Verification items for the finished model (mm, model axes). A direction names the side the tool comes from. Round coordinates to 2 decimals unless told otherwise and drop trailing zeros. Order: outer loops, then holes, each group sorted by start corner. A loop starts at its lowest first (then second) coordinate and runs counter-clockwise, first axis right, second up. Notation, with made-up numbers: M 11,-17.5 L 59,-17.5 A20 cw 59,5.5 Z; hole C 23,23.5 d6. An arc over 180 degrees is marked long. Use CSV: the item, a comma, the result in double quotes. Start each with the question number.
Q1. Gauge pin test, flat ends, axial feed: pin 1 Ø0.9 at (x, y) = (3.5, 50.5) entering from -Z; pin 2 Ø2 at (y, z) = (19, 20.5) entering from +X; pin 3 Ø1.2 at (x, z) = (1, -32.5) entering from +Y; pin 4 Ø1.8 at (y, z) = (27.5, 26.1) entering from -X. Record the tip position at first contact, or that the pin passes through.
Q2. Sectioned sample at D-D (y = 51). Enter the section's corners in (x, z), and give its area (3 significant figures).
Q3. Sectioned sample at A-A (y = 27.5). Enter the section's corners in (x, z), and give its area (4 significant figures).
Q4. Scan lines: line 1 (Y direction, x = 0.95, z = -26.1); line 2 (Z direction, x = 0.75, y = 27); line 3 (Z direction, x = 6.5, y = 44). Record each from-to range of solid material in increasing order.
Q5. Sectioned sample at B-B (z = 26.1). Enter the section's corners in (x, y).
Q6. Set-up check for faces 1 (the face through (6, 7, 18.8)), 2 (the face through (3, 48, -27.1)), 3 (the face through (1, 14.5, -33)): record each of +Z, -Z, +X, -X, +Y, -Y from which the full face is reachable in a straight line by a thin tool's end or side.
Q7. Mould release check, pull along Z, two halves, no side actions. Record for faces 4 (the face through (1, 40.5, -33)), 5 (the face through (2.5, 27, 1)), 6 (the face through (3, 7, 27.1)): +Z half, -Z half, draft (parallel to the pull), parting line (faces both ways), or undercut.
Q8. Sectioned sample at C-C (x = 5.25). Enter the section's corners in (y, z), and give its area (3 significant figures).
Autodesk Inventor part; units mm, degrees
ref_plane "YZ Plane" through (0, 0, 0) normal (1, 0, 0) x (0, 1, 0)
ref_plane "XZ Plane" through (0, 0, 0) normal (0, 1, 0) x (-1, 0, 0)
ref_plane "XY Plane" through (0, 0, 0) normal (0, 0, 1) x (1, 0, 0)
sketch "Sketch1" plane through (0, 0, 0) normal (0, 1, 0) x (-1, 0, 0)
  line L0 (0, 27.1) -> (0, -27.1)
  line L1 (0, 27.1) -> (-6.8, 27.1)
  line L2 (-6.8, 27.1) -> (-6.8, 18.8)
  line L3 (-6.8, 18.8) -> (-4.3, 18.8)
  line L4 (-4.3, 18.8) -> (-4.3, 24.6)
  line L5 (-4.3, 24.6) -> (-2.5, 24.6)
  line L6 (-2.5, 24.6) -> (-2.5, 0)
  line L7 (0, -27.1) -> (-6.8, -27.1)
  line L8 (-6.8, -27.1) -> (-6.8, -18.8)
  line L9 (-6.8, -18.8) -> (-4.3, -18.8)
  line L10 (-4.3, -18.8) -> (-4.3, -24.6)
  line L11 (-4.3, -24.6) -> (-2.5, -24.6)
  line L12 (-2.5, -24.6) -> (-2.5, 0)
  point P0 (0, 0)
  dimension "d0" = 54.2
  dimension "d1" = 6.8
  dimension "d2" = 8.3
  dimension "d3" = 2.5
  dimension "d4" = 5.8
  dimension "d5" = 1.8
  dimension "d6" = 8.3
  dimension "d7" = 5.8
extrude "Extrusion1" add sketch "Sketch1" along normal blind 14.5
sketch "Sketch2" plane through (0, 14.5, 0) normal (0, 1, 0) x (1, 0, 0)
  line L0 (2.5, -24.6) -> (2.5, 24.6)
  line L1 (2.5, 0) -> (2.5, 39.5)
  line L2 (2.5, 39.5) -> (0, 39.5)
  line L3 (0, 39.5) -> (0, 0)
  line L4 (0, 0) -> (0, -39.5)
  line L5 (0, 27.1) -> (0, -27.1)
  line L6 (0, -39.5) -> (2.5, -39.5)
  line L7 (2.5, -39.5) -> (2.5, 0)
  dimension "d10" = 39.5
  dimension "d11" = 39.5
extrude "Extrusion2" add sketch "Sketch2" along normal blind 26
sketch "Sketch3" plane through (0, 40.5, 0) normal (0, 1, 0) x (1, 0, 0)
  line L0 (2.5, -24.6) -> (2.5, 24.6)
  line L1 (2.5, 0) -> (2.5, 24.6558)
  line L2 (0, 27.1) -> (0, -27.1)
  line L3 (4.3, -24.6) -> (2.5, -24.6)
  line L4 (6.8, -18.8) -> (4.3, -18.8)
  line L5 (4.3, -24.6) -> (4.3, -18.8)
  line L6 (4.3, -18.8) -> (6.8, -18.8)
  line L7 (6.8, -18.8) -> (6.8, -27.1)
  line L8 (6.8, -27.1) -> (2.5, -27.1)
  line L9 (2.5, 0) -> (2.5, 24.6558)
  line L10 (2.5, 24.6) -> (4.3, 24.6)
  line L11 (4.3, 18.8) -> (6.8, 18.8)
  line L12 (4.3, 24.6) -> (4.3, 18.8)
  line L13 (4.3, 18.8) -> (6.8, 18.8)
  line L14 (6.8, 18.8) -> (6.8, 27.1)
  line L15 (6.8, 27.1) -> (0, 27.1)
  line L16 (0, 27.1) -> (0, -27.1)
  line L17 (6.8, -27.1) -> (0, -27.1)
  line L18 (4.3, -24.6) -> (2.5, -24.6)
  point P0 (0, 0)
extrude "Extrusion3" add sketch "Sketch3" along normal blind 14.5
sketch "Sketch4" plane through (2.5, 0, 24.6) normal (1, 0, 0) x (0, 0, -1)
  line L0 (64.1, 14.5) -> (64.1, 40.5)
  line L1 (64.1, 27.5) -> (50.7, 27.5)
  circle A0 centre (50.7, 27.5) radius 1.5
  line L2 (-14.9, 14.5) -> (-14.9, 40.5)
  line L3 (-14.9, 27.5) -> (-1.5, 27.5)
  circle A1 centre (-1.5, 27.5) radius 1.5
  point P0 (24.6, 0)
  dimension "d16" = 13.4
  dimension "d17" = 3
  dimension "d18" = 13.4
  dimension "d19" = 3
extrude "Extrusion4" cut sketch "Sketch4" against normal blind 4.5
properties part number "cam_holder2"
Verdict:
1,pin 1,"stops at z = -27.1"
1,pin 2,"stops at x = 2.5"
1,pin 3,"stops at y = 40.5"
1,pin 4,"passes through"
2,outline,"M 0,-27.1 L 6.8,-27.1 L 6.8,-18.8 L 4.3,-18.8 L 4.3,-24.6 L 2.5,-24.6 L 2.5,24.6 L 4.3,24.6 L 4.3,18.8 L 6.8,18.8 L 6.8,27.1 L 0,27.1 Z"
2,area,"186 mm²"
3,outline,"M 0,-39.5 L 2.5,-39.5 L 2.5,-27.6 L 0,-27.6 Z; M 0,-24.6 L 2.5,-24.6 L 2.5,24.6 L 0,24.6 Z; M 0,27.6 L 2.5,27.6 L 2.5,39.5 L 0,39.5 Z"
3,area,"182.5 mm²"
4,line 1,"y = 0 to 26, 29 to 55"
4,line 2,"z = -39.5 to -27.51, -24.69 to 24.69, 27.51 to 39.5"
4,line 3,"z = -27.1 to -18.8, 18.8 to 27.1"
5,outline,"M 0,0 L 6.8,0 L 6.8,14.5 L 2.5,14.5 L 2.5,26 L 0,26 Z; M 0,29 L 2.5,29 L 2.5,40.5 L 6.8,40.5 L 6.8,55 L 0,55 Z"
6,face 1,"+X, +Y, -Y"
6,face 2,"-Z, +X, -X, +Y"
6,face 3,"-Z, +X, -X, -Y"
7,face 4,"draft"
7,face 5,"undercut"
7,face 6,"+Z half"
8,outline,"M 0,-27.1 L 14.5,-27.1 L 14.5,-18.8 L 0,-18.8 Z; M 0,18.8 L 14.5,18.8 L 14.5,27.1 L 0,27.1 Z; M 40.5,-27.1 L 55,-27.1 L 55,-18.8 L 40.5,-18.8 Z; M 40.5,18.8 L 55,18.8 L 55,27.1 L 40.5,27.1 Z"
8,area,"481 mm²"
